For this review, take the finished solid that the model builds, in its own axes (mm). Coordinates: 2 decimals unless noted, no trailing zeros. Order: outer loops, then holes, each group sorted by start corner. A loop starts at its lowest first (then second) coordinate and runs counter-clockwise, first axis right, second up. Notation, with made-up numbers: M 7,74 L 17,74 A15 cw 17,78 Z; hole C 39.25,-8.75 d7. An arc over 180 degrees is marked long. Use CSV: the item, a comma, the result in double quotes.
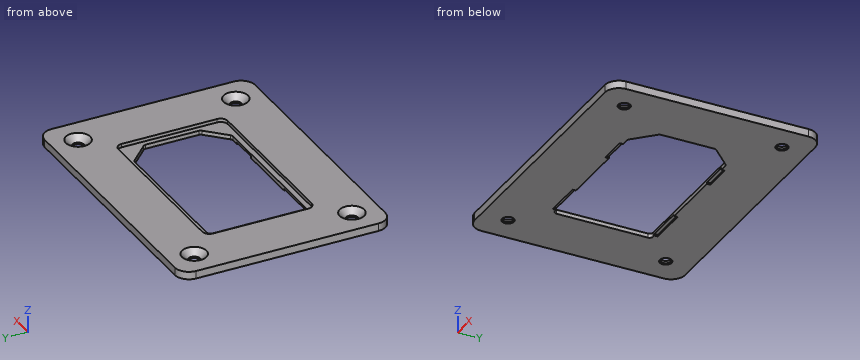
```python
from build123d import *

# Parameters (mm, degrees)
SKETCH_W        = 80
SKETCH_H        = 60
PAD_DEPTH       = 2.2
POCKET_DEPTH    = 2.201
FILLET_R        = 4
SKETCH002_R     = 1.7
POCKET001_DEPTH = 2.201
SKETCH003_W     = 50.5
SKETCH003_H     = 31.2
POCKET002_DEPTH = 1
FILLET001_R     = 2
FILLET002_R     = 1
CHAMFER_SIZE    = 1.8
SKETCH004_W     = 11
SKETCH004_H     = 1
SKETCH004_W_2   = 8
POCKET003_DEPTH = 0.5


with BuildPart() as part:
    # Sketch → Pad (new body)
    with BuildSketch(Plane.XY):
        Rectangle(SKETCH_W, SKETCH_H)
    extrude(amount=PAD_DEPTH)

    # Sketch001 → Pocket (cut, through all)
    with BuildSketch(Plane.XY.offset(2.2)):
        Polygon((-23.65, 14), (17.65, 14), (23.65, 8), (23.65, -8), (17.65, -14), (-23.65, -14), align=None)
    extrude(amount=-POCKET_DEPTH, mode=Mode.SUBTRACT)

    # Fillet
    fillet_edges = [part.edges().sort_by_distance(p)[0] for p in [
        (-40, -30, 1.1),
        (-40, 30, 1.1),
        (40, -30, 1.1),
        (40, 30, 1.1),
    ]]
    fillet(fillet_edges, radius=FILLET_R)

    # Sketch002 → Pocket001 (cut, through all)
    with BuildSketch(Plane.XY.offset(2.2)):
        with Locations((-32.135281, 22.485281)):
            Circle(SKETCH002_R)
        with Locations((32.135281, 22.485281)):
            Circle(SKETCH002_R)
        with Locations((32.135281, -22.485281)):
            Circle(SKETCH002_R)
        with Locations((-32.135281, -22.485281)):
            Circle(SKETCH002_R)
    extrude(amount=-POCKET001_DEPTH, mode=Mode.SUBTRACT)

    # Sketch003 → Pocket002 (cut)
    with BuildSketch(Plane.XY.offset(2.2)):
        Rectangle(SKETCH003_W, SKETCH003_H)
    extrude(amount=-POCKET002_DEPTH, mode=Mode.SUBTRACT)

    # Fillet001
    fillet001_edges = [part.edges().sort_by_distance(p)[0] for p in [
        (-25.25, -15.6, 1.7),
        (25.25, -15.6, 1.7),
        (-25.25, 15.6, 1.7),
        (25.25, 15.6, 1.7),
    ]]
    fillet(fillet001_edges, radius=FILLET001_R)

    # Fillet002
    fillet002_edges = [part.edges().sort_by_distance(p)[0] for p in [
        (17.65, -14, 0.6),
        (-23.65, -14, 0.6),
        (23.65, -8, 0.6),
        (23.65, 8, 0.6),
        (-23.65, 14, 0.6),
        (17.65, 14, 0.6),
    ]]
    fillet(fillet002_edges, radius=FILLET002_R)

    # Chamfer
    chamfer_edges = [part.edges().sort_by_distance(p)[0] for p in [
        (-33.835281, 22.485281, 2.2),
        (30.435281, 22.485281, 2.2),
        (30.435281, -22.485281, 2.2),
        (-33.835281, -22.485281, 2.2),
    ]]
    chamfer(chamfer_edges, length=CHAMFER_SIZE)

    # Sketch004 → Pocket003 (cut)
    with BuildSketch(Plane(origin=(0, 0, 0), x_dir=(1, 0, 0), z_dir=(0, 0, -1))):
        with Locations((-16.51054, 14.48414)):
            Rectangle(SKETCH004_W, SKETCH004_H)
        with Locations((-16.51054, -14.479152)):
            Rectangle(SKETCH004_W, SKETCH004_H)
        with Locations((11.1315, 14.48414)):
            Rectangle(SKETCH004_W_2, SKETCH004_H)
        with Locations((11.1315, -14.479152)):
            Rectangle(SKETCH004_W_2, SKETCH004_H)
    extrude(amount=-POCKET003_DEPTH, mode=Mode.SUBTRACT)


solid = part.part
```
Item 1: Add section B-B on y = 3.5. State the section outline as (x, z) points.
Solutions:
outline,"M -40,0 L -23.65,0 L -23.65,1.2 L -25.25,1.2 L -25.25,2.2 L -40,2.2 Z; M 23.65,0 L 40,0 L 40,2.2 L 25.25,2.2 L 25.25,1.2 L 23.65,1.2 Z"
Item 2: Clearance check with flat-ended pins moving along their axes: pin 1 Ø3 at (x, y) = (32.14, 22.49) entering from +Z; pin 2 Ø0.5 at (x, y) = (12, 14.5) entering from -Z. State where each tip first meets the part, or that it passes through.
Solutions:
pin 1,"through"
pin 2,"z = 0.5"
Item 3: Add section C-C on z = 1.8. State the section outline as (x, y) points.
Solutions:
outline,"M -40,-26 A4 ccw -36,-30 L 36,-30 A4 ccw 40,-26 L 40,26 A4 ccw 36,30 L -36,30 A4 ccw -40,26 Z; hole C -32.14,-22.49 d6.2; hole C -32.14,22.49 d6.2; hole M -25.25,-13.6 A2 ccw -23.25,-15.6 L 23.25,-15.6 A2 ccw 25.25,-13.6 L 25.25,13.6 A2 ccw 23.25,15.6 L -23.25,15.6 A2 ccw -25.25,13.6 Z; hole C 32.14,-22.49 d6.2; hole C 32.14,22.49 d6.2"
Item 4: To check wall thickness, follow line 1 along X through (y, z) = (-12.5, 1.35); line 2 along Y through (x, z) = (1.5, 0.45); line 3 along X through (y, z) = (-5.5, 0.2). State the ranges of each line that lie inside material, in increasing order. Write a range as [from, to].
Solutions:
line 1,"[-40, -25.25], [25.25, 40]"
line 2,"[-30, -14], [14, 30]"
line 3,"[-40, -23.65], [23.65, 40]"
Item 5: Add section A-A on x = -19. State the section outline as (y, z) points.
Solutions:
outline,"M -30,0 L -14.98,0 L -14.98,0.5 L -14,0.5 L -14,1.2 L -15.6,1.2 L -15.6,2.2 L -30,2.2 Z; M 14,0.5 L 14.98,0.5 L 14.98,0 L 30,0 L 30,2.2 L 15.6,2.2 L 15.6,1.2 L 14,1.2 Z"
